Read the model definition and answer for the solid it produces. Units are mm, in the model's axes. Face numbers are marked on the shaded views. A direction names the side the tool comes from. Coordinates: 2 decimals unless noted, no trailing zeros. Write each loop counter-clockwise with the first axis right and the second up, starting at its lowest first coordinate (ties: lowest second). Pieces come first, ordered by that corner, then holes. Notation, with made-up numbers: (7, 57) -> (31, 57) arc R23 ccw to (31, 75) -> close; hole circle Ø6 at (26, 34.5). An arc over 180 degrees is marked (long way). Return JSON: item names as keys, results as strings.
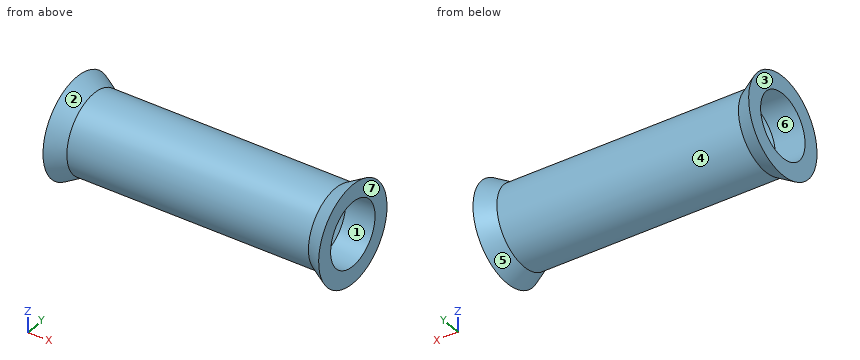
from build123d import *

# Parameters (mm, degrees)
SKETCH1_W = 30
SKETCH1_H = 4
SKETCH2_W = 2
SKETCH2_H = 5


with BuildPart() as part:
    # Sketch1 → Base-Revolve (revolve)
    with BuildSketch(Plane.XY, mode=Mode.PRIVATE) as base_revolve_sk:
        with Locations((0, 2)):
            Rectangle(SKETCH1_W, SKETCH1_H)
    revolve(base_revolve_sk.sketch.rotate(Axis((-30, 0, 0), (1, 0, 0)), 90), axis=Axis((-30, 0, 0), (1, 0, 0)))

    # Sketch2 → Cut-to-GripLength (revolve, cut)
    with BuildSketch(Plane.XY):
        with Locations((-15, 2.5)):
            Rectangle(SKETCH2_W, SKETCH2_H)
        with Locations((15, 2.5)):
            Rectangle(SKETCH2_W, SKETCH2_H)
    revolve(axis=Axis((-30, 0, 0), (1, 0, 0)), mode=Mode.SUBTRACT)

    # Sketch4 → HeadTypeB (revolve)
    with BuildSketch(Plane.XY, mode=Mode.PRIVATE) as headtypeb_sk:
        Polygon((-14, 0), (-14, 5), (-12.267949192, 4), (-12.267949192, 0), align=None)
        Polygon((12.267949192, 0), (14, 0), (14, 5), (12.267949192, 4), align=None)
    revolve(headtypeb_sk.sketch.rotate(Axis((-20, 0, 0), (1, 0, 0)), 90), axis=Axis((-20, 0, 0), (1, 0, 0)))

    # Sketch5 → HoleTypeA (revolve, cut)
    with BuildSketch(Plane.XY, mode=Mode.PRIVATE) as holetypea_sk:
        Polygon((-9.123611625, 0), (-11, 3.25), (-15, 3.25), (-15, 0), align=None)
        Polygon((9.123611625, 0), (11, 3.25), (15, 3.25), (15, 0), align=None)
    revolve(holetypea_sk.sketch.rotate(Axis((-22, 0, 0), (1, 0, 0)), 90), axis=Axis((-22, 0, 0), (1, 0, 0)), mode=Mode.SUBTRACT)


solid = part.part
1. Flat-ended cylindrical pins translate along their axes: pin 1 Ø1 at (x, y) = (-6.5, -1) entering from +Z; pin 2 Ø5 at (y, z) = (0, 0) entering from +X; pin 3 Ø3 at (x, z) = (-3, -3.5) entering from +Y. Find the tip coordinate at first contact, or state that the pin passes through.
Taken from the geometry:
{"pin 1": "stops at z = 3.97", "pin 2": "stops at x = 10.57", "pin 3": "stops at y = 3.46"}
2. For a pull along X with two mould halves and no side action, classify the marked faces 4, 5, 6 and 7 as +X half, -X half, draft (parallel to the pull), parting line (faces both ways), or undercut.
Taken from the geometry:
{"face 4": "undercut", "face 5": "undercut", "face 6": "draft", "face 7": "+X half"}
3. The part is cut by section A-A (x = 4.75). Determine the outline of the cut face in (y, z).
Taken from the geometry:
{"outline": "circle Ø8 at (0, 0)"}
4. Consider L1, parallel to Y at x = -11.9, z = 0; L2, parallel to Y at x = -13.4, z = 0; L3, parallel to X at y = -3.25, z = 2.5. Determine where each line is inside the solid, lowest interval first.
Taken from the geometry:
{"L1": "y = -4 to -3.25, 3.25 to 4", "L2": "y = -4.65 to -3.25, 3.25 to 4.65", "L3": "x = -14 to -12.44, 12.44 to 14"}
5. A tool of negligible diameter and unlimited length cuts with its end or side. For the marked faces 1, 2 and 3, from which of +Z, -Z, +X, -X, +Y, -Y can it reach the whole face along a straight path? Write none if from no direction.
Taken from the geometry:
{"face 1": "+X", "face 2": "none", "face 3": "+Z, -Z, -X, +Y, -Y"}
